Source: CAD feature listing. Evaluate the final solid. Frame: model axes, mm. Face numbers are marked on the shaded views. A direction names the side the tool comes from. Give positions to 0.01 mm unless a question says otherwise; leave off trailing zeros. Order: outer loops, then holes, each group sorted by start corner. A loop starts at its lowest first (then second) coordinate and runs counter-clockwise, first axis right, second up.
from build123d import *

# Parameters (mm, degrees)
BOSS_EXTRUDE1_DEPTH = 28
CUT_EXTRUDE1_DEPTH  = 5
SKETCH3_R           = 2.5
BOSS_EXTRUDE2_DEPTH = 6
SKETCH4_R           = 1.5
BOSS_EXTRUDE3_DEPTH = 5


with BuildPart() as part:
    # Sketch1 → Boss-Extrude1 (new body)
    with BuildSketch(Plane.XY):
        with BuildLine():
            Line((2.2, -3.15), (-2.2, -3.15))
            ThreePointArc((-2.2, -3.15), (-5.35, 0), (-2.2, 3.15))
            Line((-2.2, 3.15), (2.2, 3.15))
            ThreePointArc((2.2, 3.15), (5.35, 0), (2.2, -3.15))
        make_face()
    extrude(amount=-BOSS_EXTRUDE1_DEPTH)

    # Sketch1<3> → Cut-Extrude1 (cut)
    with BuildSketch(Plane.XY):
        with BuildLine():
            Line((2.85, -1.35), (-2.85, -1.35))
            ThreePointArc((-2.85, -1.35), (-4.2, 0), (-2.85, 1.35))
            Line((-2.85, 1.35), (2.85, 1.35))
            ThreePointArc((2.85, 1.35), (4.2, 0), (2.85, -1.35))
        make_face()
    extrude(amount=-CUT_EXTRUDE1_DEPTH, mode=Mode.SUBTRACT)

    # Sketch3 → Boss-Extrude2 (add)
    with BuildSketch(Plane(origin=(0, 0, -28), x_dir=(-1, 0, 0), z_dir=(0, 0, -1))):
        Circle(SKETCH3_R)
    extrude(amount=BOSS_EXTRUDE2_DEPTH)

    # Sketch4 → Boss-Extrude3 (add)
    with BuildSketch(Plane(origin=(0, 0, -34), x_dir=(-1, 0, 0), z_dir=(0, 0, -1))):
        Circle(SKETCH4_R)
    extrude(amount=BOSS_EXTRUDE3_DEPTH)


solid = part.part
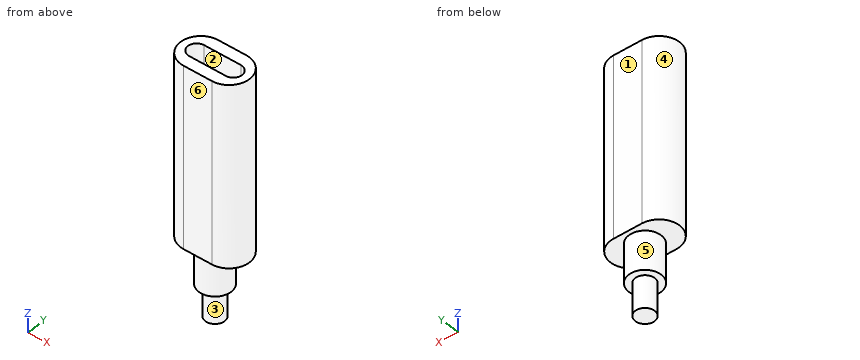
1) First-contact query: pin 1 Ø2 at (y, z) = (-1.5, -17.5) entering from -X; pin 2 Ø2 at (y, z) = (1.5, -7) entering from +X. Flat tips, straight axial feed; report the tip coordinate or a pass-through.
Checks:
pin 1: stops at x = -5.31
pin 2: stops at x = 5.31
2) Ray query, L1, parallel to Z at x = 4.5, y = 2; L2, parallel to X at y = -0.25, z = -4; L3, parallel to Z at x = 1, y = 1.75. Return the intervals inside material, ascending.
Checks:
L1: z = -28 to 0
L2: x = -5.34 to -4.18, 4.18 to 5.34
L3: z = -34 to 0
3) Section query C-C on x = 0. Output: boundary loops of the cut face in (y, z).
Checks:
outline: (-3.15, -28) - (-2.5, -28) - (-2.5, -34) - (-1.5, -34) - (-1.5, -39) - (1.5, -39) - (1.5, -34) - (2.5, -34) - (2.5, -28) - (3.15, -28) - (3.15, 0) - (1.35, 0) - (1.35, -5) - (-1.35, -5) - (-1.35, 0) - (-3.15, 0) - close
4) Section query D-D on z = -36. Output: boundary loops of the cut face in (x, y).
Checks:
outline: circle Ø3 at (0, 0)
5) Reachability of the marked faces 5 and 6 from +Z, -Z, +X, -X, +Y, -Y: full face, straight path, thin tool, end or side. Return the list, or none.
Checks:
face 5: -Z
face 6: +Z, -Z, +X, -X, -Y
6) Section query A-A on z = -4.5. Output: boundary loops of the cut face in (x, y).
Checks:
outline: (-2.2, -3.15) - (2.2, -3.15) arc R3.15 ccw to (2.2, 3.15) - (-2.2, 3.15) arc R3.15 ccw to start; hole (-2.85, -1.35) - (2.85, -1.35) arc R1.35 ccw to (2.85, 1.35) - (-2.85, 1.35) arc R1.35 ccw to start
7) Section query B-B on y = 0. Output: boundary loops of the cut face in (x, z), and give its area (3 significant figures).
Checks:
outline: (-5.35, -28) - (-2.5, -28) - (-2.5, -34) - (-1.5, -34) - (-1.5, -39) - (1.5, -39) - (1.5, -34) - (2.5, -34) - (2.5, -28) - (5.35, -28) - (5.35, 0) - (4.2, 0) - (4.2, -5) - (-4.2, -5) - (-4.2, 0) - (-5.35, 0) - close
area: 303 mm2
8) Pull-direction query (X, two-part tool) for the marked faces 1, 2, 3 and 4; classes: +X half, -X half, draft (parallel to the pull), parting line (faces both ways), or undercut.
Checks:
face 1: draft
face 2: undercut
face 3: parting line
face 4: -X half
